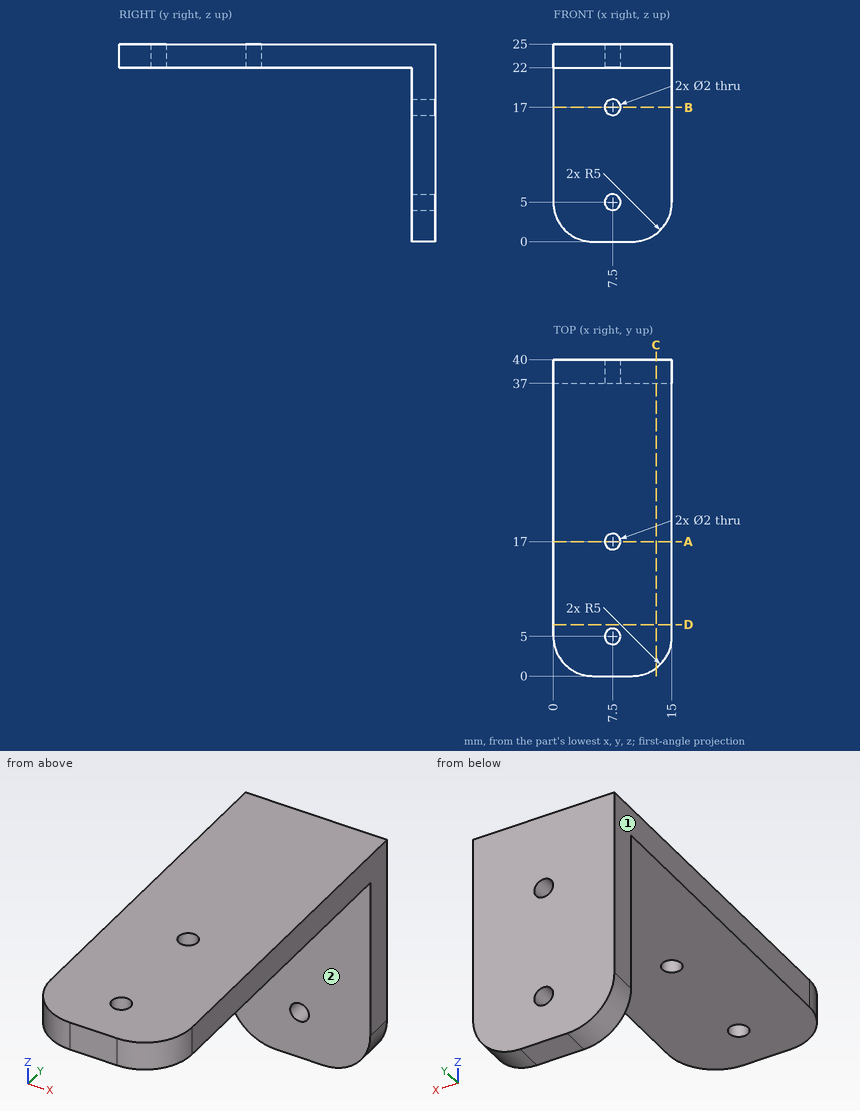
Check sheet for the drawn part. Datum: minimum x, y, z corner. Units: mm. A direction names the side the tool comes from. Round coordinates to 2 decimals unless told otherwise and drop trailing zeros. Order: outer loops, then holes, each group sorted by start corner. A loop starts at its lowest first (then second) coordinate and runs counter-clockwise, first axis right, second up.
1. Section check B-B on z = 17. Record the cut outline in (x, y), then the cut area to 3 significant figures.
Final values:
outline: (0, 37) - (6.5, 37) - (6.5, 40) - (0, 40) - close; (8.5, 37) - (15, 37) - (15, 40) - (8.5, 40) - close
area: 39.0 mm2
2. Go/stop test with flat-tipped pins: P1, Ø1, axis at y = 17.5, z = 21, coming from the -X side; P2, Ø4.5, axis at x = 6.5, y = 18.5, coming from the -Z side; P3, Ø2, axis at x = 5.5, z = 7.5, coming from the -Y side. Record where each tip stops, or that it passes through.
Final values:
P1: passes through
P2: stops at z = 22
P3: stops at y = 37
3. Section check C-C on x = 13. Record the cut outline in (y, z), then the cut area to 3 significant figures.
Final values:
outline: (1, 22) - (37, 22) - (37, 1) - (40, 1) - (40, 25) - (1, 25) - close
area: 180 mm2
4. Thickness scan on L1, parallel to Z at x = 7.5, y = 38; L2, parallel to Y at x = 7.5, z = 23.65; L3, parallel to X at y = 37.7, z = 17. Record the ranges inside material, lowest first.
Final values:
L1: z = 0 to 4, 6 to 16, 18 to 25
L2: y = 0 to 4, 6 to 16, 18 to 40
L3: x = 0 to 6.5, 8.5 to 15
5. Access from +Z, -Z, +X, -X, +Y, -Y to the whole of each face (thin tool, end or side, straight path). Record for the marked faces 1 and 2.
Final values:
face 1: +Z, -Z, -X, +Y, -Y
face 2: -Z, +X, -X, -Y
6. Section check A-A on y = 17. Record the cut outline in (x, z), then the cut area to 3 significant figures.
Final values:
outline: (0, 22) - (6.5, 22) - (6.5, 25) - (0, 25) - close; (8.5, 22) - (15, 22) - (15, 25) - (8.5, 25) - close
area: 39.0 mm2
7. Section check D-D on y = 6.5. Record the cut outline in (x, z), then the cut area to 3 significant figures.
Final values:
outline: (0, 22) - (15, 22) - (15, 25) - (0, 25) - close
area: 45.0 mm2
